Part print with two shaded views. Sizes in mm from the minimum x, y, z corner. A direction names the side the tool comes from. Coordinates: 2 decimals unless noted, no trailing zeros. Order: outer loops, then holes, each group sorted by start corner. A loop starts at its lowest first (then second) coordinate and runs counter-clockwise, first axis right, second up.
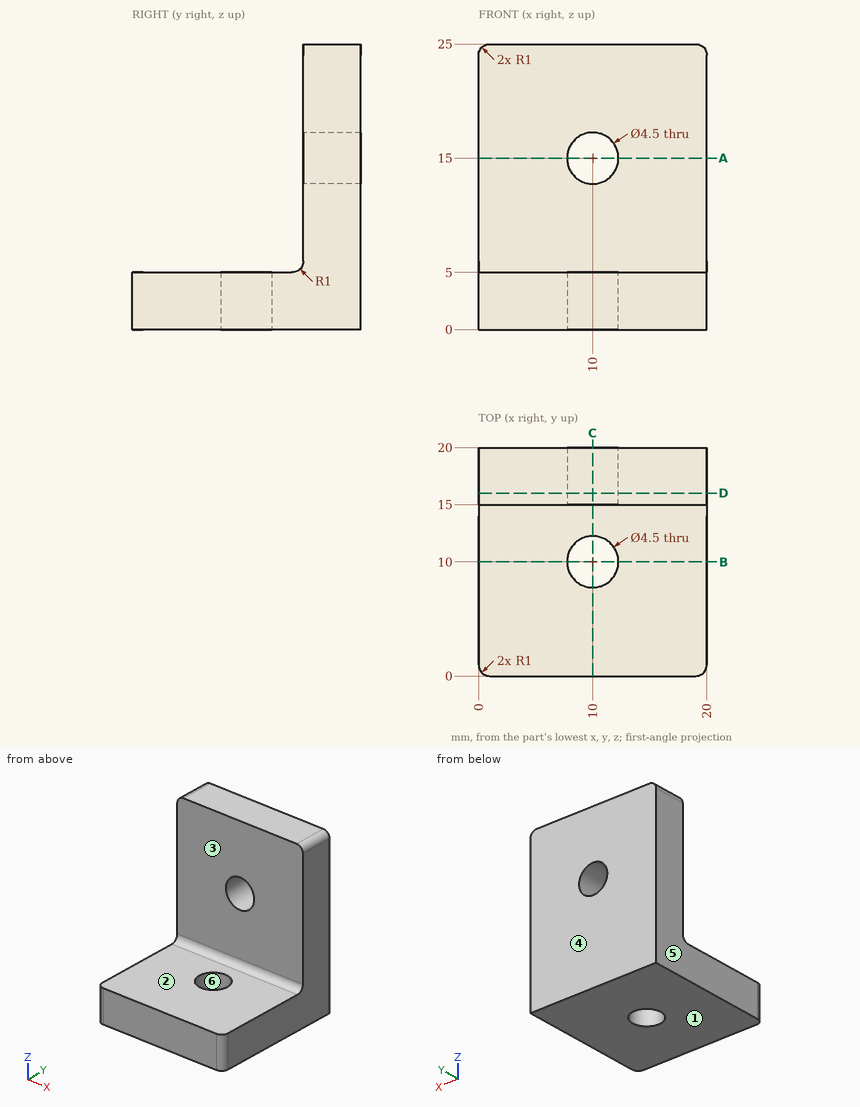
Q1. Pin check, flat tips, straight feed: pin 1 Ø8 at (x, y) = (4.5, 5) entering from +Z; pin 2 Ø4 at (x, y) = (10, 10) entering from -Z; pin 3 Ø11 at (x, y) = (12, 9) entering from +Z; pin 4 Ø5.5 at (x, z) = (7.5, 19.5) entering from -Y. Stop position of each tip, or through.
Results list:
pin 1: stops at z = 5
pin 2: passes through
pin 3: stops at z = 5.13
pin 4: stops at y = 15
Q2. Cut at D-D on y = 16. Write the cut outline in (x, z).
Results list:
outline: (0, 0) - (20, 0) - (20, 24) arc R1 ccw to (19, 25) - (1, 25) arc R1 ccw to (0, 24) - close; hole circle Ø4.5 at (10, 15)
Q3. Cut at B-B on y = 10. Write the cut outline in (x, z), and give its area (3 significant figures).
Results list:
outline: (0, 0) - (7.75, 0) - (7.75, 5) - (0, 5) - close; (12.25, 0) - (20, 0) - (20, 5) - (12.25, 5) - close
area: 77.5 mm2
Q4. Which spindle directions (+Z, -Z, +X, -X, +Y, -Y) get a long thin tool onto all of the face, cutting with end or side? Do the marked faces 1 and 2. Say none if no direction does.
Results list:
face 1: -Z, +X, -X, +Y, -Y
face 2: +Z, +X, -X, -Y
Q5. Wall check: line 1 along Z through (x, y) = (10, 17.2); line 2 along Y through (x, z) = (10, 2.4); line 3 along Y through (x, z) = (17.75, 13.25). Give the ranges that are in metal, low to high.
Results list:
line 1: z = 0 to 12.75, 17.25 to 25
line 2: y = 0 to 7.75, 12.25 to 20
line 3: y = 15 to 20
Q6. Cut at A-A on z = 15. Write the cut outline in (x, y), and give its area (3 significant figures).
Results list:
outline: (0, 15) - (7.75, 15) - (7.75, 20) - (0, 20) - close; (12.25, 15) - (20, 15) - (20, 20) - (12.25, 20) - close
area: 77.5 mm2
Q7. Cut at C-C on x = 10. Write the cut outline in (y, z).
Results list:
outline: (0, 0) - (7.75, 0) - (7.75, 5) - (0, 5) - close; (12.25, 0) - (20, 0) - (20, 12.75) - (15, 12.75) - (15, 6) arc R1 cw to (14, 5) - (12.25, 5) - close; (15, 17.25) - (20, 17.25) - (20, 25) - (15, 25) - close
Q8. Mould opens along Y. For the marked faces 3, 4, 5 and 6 say: pulls with the +Y half, pulls with the -Y half, needs draft (parallel to the pull), parting line crosses it, or undercut.
Results list:
face 3: pulls with the -Y half
face 4: pulls with the +Y half
face 5: needs draft
face 6: undercut
